from build123d import *

# Parameters (mm, degrees)
SKETCH1_R           = 1.720095417
SKETCH1_R_2         = 1.632335783
SKETCH1_R_3         = 1.27
BOSS_EXTRUDE1_DEPTH = 2.54


with BuildPart() as part:
    # Sketch1 → Boss-Extrude1 (new body)
    with BuildSketch(Plane.XY):
        with BuildLine():
            Line((0.359622665, 84.647626996), (0.359622665, 112.547896558))
            ThreePointArc((0.359622665, 112.547896558), (1.569792033, 115.17822767), (4.285435965, 116.18243367))
            Line((4.285435965, 116.18243367), (699.960441306, 116.18243367))
            Line((699.960441306, 116.18243367), (699.960441306, 131.904163347))
            ThreePointArc((699.960441306, 131.904163347), (701.183091811, 134.700225562), (704.024750828, 135.812795653))
            Line((704.024750828, 135.812795653), (946.192785632, 135.812795653))
            ThreePointArc((946.192785632, 135.812795653), (948.657072186, 134.878542119), (949.738968911, 132.475411377))
            Line((949.738968911, 132.475411377), (949.738968911, 64.012598058))
            ThreePointArc((949.738968911, 64.012598058), (948.74540471, 61.39621374), (946.192785632, 60.24870663))
            Line((946.192785632, 60.24870663), (704.024750828, 60.24870663))
            ThreePointArc((704.024750828, 60.24870663), (701.213068629, 61.288906282), (699.960441306, 64.012598058))
            Line((699.960441306, 64.012598058), (699.960441306, 81.011908201))
            Line((699.960441306, 81.011908201), (4.285435965, 81.011908201))
            ThreePointArc((4.285435965, 81.011908201), (1.569547298, 82.016705042), (0.359622665, 84.647626996))
        make_face()
        with Locations((94.1622142, 88.091107164)):
            Circle(SKETCH1_R, mode=Mode.SUBTRACT)
        with Locations((94.1622142, 108.484732819)):
            Circle(SKETCH1_R, mode=Mode.SUBTRACT)
        with Locations((221.392126764, 108.484732819)):
            Circle(SKETCH1_R, mode=Mode.SUBTRACT)
        with Locations((221.392126764, 88.091107164)):
            Circle(SKETCH1_R, mode=Mode.SUBTRACT)
        with Locations((348.078760153, 108.484732819)):
            Circle(SKETCH1_R, mode=Mode.SUBTRACT)
        with Locations((348.078760153, 88.091107164)):
            Circle(SKETCH1_R_2, mode=Mode.SUBTRACT)
        with Locations((475.146430575, 108.484732819)):
            Circle(SKETCH1_R, mode=Mode.SUBTRACT)
        with Locations((475.146430575, 88.091107164)):
            Circle(SKETCH1_R, mode=Mode.SUBTRACT)
        with Locations((602.130384222, 88.091107164)):
            Circle(SKETCH1_R, mode=Mode.SUBTRACT)
        with Locations((602.130384222, 108.484732819)):
            Circle(SKETCH1_R, mode=Mode.SUBTRACT)
        with Locations((705.892847696, 116.18243367)):
            Circle(SKETCH1_R_3, mode=Mode.SUBTRACT)
        with Locations((705.892847696, 81.011908201)):
            Circle(SKETCH1_R_3, mode=Mode.SUBTRACT)
        with Locations((760.070975046, 130.611938178)):
            Circle(SKETCH1_R_3, mode=Mode.SUBTRACT)
        with Locations((760.070975046, 66.505299661)):
            Circle(SKETCH1_R_3, mode=Mode.SUBTRACT)
        with Locations((848.138968911, 130.611938178)):
            Circle(SKETCH1_R_3, mode=Mode.SUBTRACT)
        with Locations((848.138968911, 66.505299661)):
            Circle(SKETCH1_R_3, mode=Mode.SUBTRACT)
        with Locations((943.890172073, 116.18243367)):
            Circle(SKETCH1_R_3, mode=Mode.SUBTRACT)
        with Locations((943.890172073, 81.011908201)):
            Circle(SKETCH1_R_3, mode=Mode.SUBTRACT)
    extrude(amount=BOSS_EXTRUDE1_DEPTH)


solid = part.part
Geometry: final body of the model. Coordinates: model frame, mm. Coordinates: 2 decimals unless noted, no trailing zeros. Order: outer loops, then holes, each group sorted by start corner. A loop starts at its lowest first (then second) coordinate and runs counter-clockwise, first axis right, second up.
(1) First-contact query: pin 1 (1.3 mm diameter, centred on x = 841, z = 1, fed in from -Y); pin 2 (8 mm diameter, centred on x = 102.5, y = 86, fed in from -Z); pin 3 (3 mm diameter, centred on x = 94.16, y = 88.09, fed in from +Z); pin 4 (1.3 mm diameter, centred on y = 74, z = 2, fed in from -X). Flat tips, straight axial feed; report the tip coordinate or a pass-through.
(2) Material intervals for probe 1 along X at (y, z) = (81.5, 1.5); probe 2 along X at (y, z) = (110, 1.45); probe 3 along Y at (x, z) = (378.5, 1.2), sorted ascending.
(3) Section query B-B (x = 281.5). Return the cut outline in (y, z).
(4) Section query A-A (z = 0.95). State how many separate pieces and enclosed holes the cut face has, plus the area to 3 significant figures.
Solution:
1. pin 1: stops at y = 60.25
1. pin 2: stops at z = 0
1. pin 3: passes through
1. pin 4: stops at x = 699.96
2. probe 1: x = 2.28 to 704.72, 707.07 to 942.72, 945.06 to 949.74
2. probe 2: x = 0.36 to 93.35, 94.98 to 220.58, 222.21 to 347.26, 348.89 to 474.33, 475.96 to 601.32, 602.94 to 949.74
2. probe 3: y = 81.01 to 116.18
3. outline: (81.01, 0) - (116.18, 0) - (116.18, 2.54) - (81.01, 2.54) - close
4. separate pieces: 1
4. enclosed holes: 18
4. area: 43,300 mm2
